Part model, mm, in its own coordinate system. Give positions to 0.01 mm unless a question says otherwise; leave off trailing zeros. Write each loop counter-clockwise with the first axis right and the second up, starting at its lowest first coordinate (ties: lowest second). Pieces come first, ordered by that corner, then holes.
Autodesk Inventor part; units mm, degrees
ref_plane "YZ Plane" through (0, 0, 0) normal (1, 0, 0) x (0, 1, 0)
ref_plane "XZ Plane" through (0, 0, 0) normal (0, 1, 0) x (-1, 0, 0)
ref_plane "XY Plane" through (0, 0, 0) normal (0, 0, 1) x (1, 0, 0)
sketch "Sketch1" plane through (0, 0, 0) normal (0, 1, 0) x (-1, 0, 0)
  line L0 (0, 0) -> (685.8, 0)
  line L1 (685.8, 0) -> (685.8, -584.2)
  line L2 (685.8, -584.2) -> (0, -584.2)
  line L3 (0, -584.2) -> (0, 0)
  dimension "d0" = 685.8
  dimension "d1" = 584.2
extrude "Extrusion1" add sketch "Sketch1" along normal blind 12.7
sketch "Sketch2" plane through (0, 12.7, 0) normal (0, 1, 0) x (1, 0, 0)
  line L0 (-436.88, 0) -> (-248.92, 0)
  line L1 (-248.92, 0) -> (-248.92, 234.95)
  line L2 (-248.92, 234.95) -> (-436.88, 234.95)
  line L3 (-436.88, 234.95) -> (-436.88, 0)
  line L4 (0, 584.2) -> (-685.8, 584.2)
  line L5 (-436.88, 584.2) -> (-248.92, 584.2)
  line L6 (-248.92, 584.2) -> (-248.92, 349.25)
  line L7 (-248.92, 349.25) -> (-436.88, 349.25)
  line L8 (-436.88, 349.25) -> (-436.88, 584.2)
  line L9 (-685.8, 0) -> (0, 0)
  line L10 (-436.88, 349.25) -> (-436.88, 234.95) construction
  line L11 (-685.8, 584.2) -> (-685.8, 0) construction
  point P0 (-342.9, 0)
  point P1 (-342.9, 0)
  point P2 (-342.9, 0)
  point P3 (-342.9, 584.2)
  point P4 (-342.9, 584.2)
  point P5 (-436.88, 292.1)
  point P6 (-685.8, 292.1)
  dimension "d4" = 187.96
  dimension "d6" = 187.96
  dimension "d10" = 114.3
extrude "Extrusion2" cut sketch "Sketch2" against normal through all
sketch "Sketch3" plane through (0, 12.7, 0) normal (0, 1, 0) x (1, 0, 0)
  line L0 (0, 0) -> (0, 584.2)
  line L1 (0, 0) -> (-127, 0)
  line L2 (-127, 0) -> (-127, 63.5)
  line L3 (-127, 63.5) -> (0, 63.5)
  line L4 (0, 63.5) -> (0, 0)
  line L5 (0, 584.2) -> (-127, 584.2)
  line L6 (-127, 584.2) -> (-127, 520.7)
  line L7 (-127, 520.7) -> (0, 520.7)
  line L8 (0, 520.7) -> (0, 584.2)
  line L9 (-685.8, 584.2) -> (-558.8, 584.2)
  line L10 (-558.8, 584.2) -> (-558.8, 520.7)
  line L11 (-558.8, 520.7) -> (-685.8, 520.7)
  line L12 (-685.8, 520.7) -> (-685.8, 584.2)
  line L13 (-685.8, 0) -> (-558.8, 0)
  line L14 (-558.8, 0) -> (-558.8, 63.5)
  line L15 (-558.8, 63.5) -> (-685.8, 63.5)
  line L16 (-685.8, 63.5) -> (-685.8, 0)
  dimension "d11" = 127
  dimension "d12" = 63.5
  dimension "d13" = 127
  dimension "d14" = 63.5
  dimension "d15" = 127
  dimension "d16" = 63.5
  dimension "d17" = 127
  dimension "d18" = 63.5
extrude "Extrusion3" cut sketch "Sketch3" against normal through all
properties part number "base board" material "Wood (Birch)"
1) Saw through at D-D, the plane x = -283. Write the cut outline in (y, z).
Answers follow:
outline: (0, -349.25) - (12.7, -349.25) - (12.7, -234.95) - (0, -234.95) - close
2) Wall check: L1, parallel to X at y = 7, z = -119.5; L2, parallel to X at y = 5, z = -62.5; L3, parallel to Z at x = -71.5, y = 2.5. Give the ranges that are in metal, low to high.
Answers follow:
L1: x = -685.8 to -436.88, -248.92 to 0
L2: x = -558.8 to -436.88, -248.92 to -127
L3: z = -520.7 to -63.5
3) Saw through at A-A, the plane z = -476. Write the cut outline in (x, y).
Answers follow:
outline: (-685.8, 0) - (-436.88, 0) - (-436.88, 12.7) - (-685.8, 12.7) - close; (-248.92, 0) - (0, 0) - (0, 12.7) - (-248.92, 12.7) - close
4) Saw through at C-C, the plane z = -542. Write the cut outline in (x, y).
Answers follow:
outline: (-558.8, 0) - (-436.88, 0) - (-436.88, 12.7) - (-558.8, 12.7) - close; (-248.92, 0) - (-127, 0) - (-127, 12.7) - (-248.92, 12.7) - close
5) Saw through at B-B, the plane y = 8. Write the cut outline in (x, z).
Answers follow:
outline: (-685.8, -520.7) - (-558.8, -520.7) - (-558.8, -584.2) - (-436.88, -584.2) - (-436.88, -349.25) - (-248.92, -349.25) - (-248.92, -584.2) - (-127, -584.2) - (-127, -520.7) - (0, -520.7) - (0, -63.5) - (-127, -63.5) - (-127, 0) - (-248.92, 0) - (-248.92, -234.95) - (-436.88, -234.95) - (-436.88, 0) - (-558.8, 0) - (-558.8, -63.5) - (-685.8, -63.5) - close
6) Pin check, flat tips, straight feed: pin 1 Ø4 at (y, z) = (9, -475.5) entering from +X; pin 2 Ø4 at (x, y) = (-604.5, 9) entering from +Z; pin 3 Ø4 at (x, y) = (-324, 6.5) entering from -Z; pin 4 Ø4 at (y, z) = (8.5, -26.5) entering from -X. Stop position of each tip, or through.
Answers follow:
pin 1: stops at x = 0
pin 2: stops at z = -63.5
pin 3: stops at z = -349.25
pin 4: stops at x = -558.8
